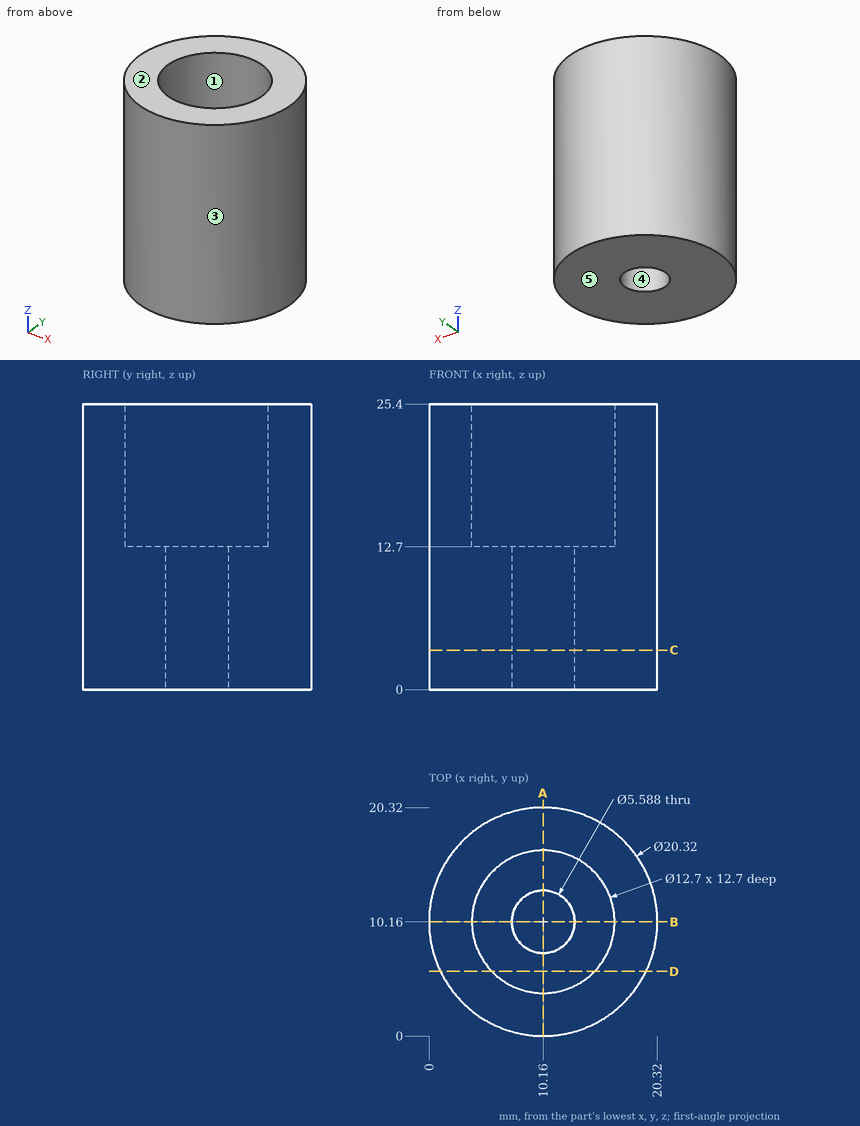
Part print with two shaded views. Sizes in mm from the minimum x, y, z corner. A direction names the side the tool comes from. Coordinates: 2 decimals unless noted, no trailing zeros. Write each loop counter-clockwise with the first axis right and the second up, starting at its lowest first coordinate (ties: lowest second). Pieces come first, ordered by that corner, then holes.
(1) Drill centre lines: line 1 (Y direction, x = 10.16, z = 22.5); line 2 (Y direction, x = 10.16, z = 3.25); line 3 (X direction, y = 10.5, z = 4.25). Where is each one in solid material? Low to high.
(2) Pin check, flat tips, straight feed: pin 1 Ø3 at (x, z) = (16.5, 13) entering from -Y; pin 2 Ø3.5 at (x, y) = (10.16, 10.16) entering from -Z; pin 3 Ø12 at (x, y) = (9.5, 14) entering from +Z; pin 4 Ø3 at (x, z) = (17, 11.5) entering from +Y. Stop position of each tip, or through.
(3) Cut at C-C on z = 3.5. List the corners of the cut face in (x, y), and give its area (3 significant figures).
(4) 3-axis set-ups, long thin cutter, end or side, ignore diameter. For the marked faces 1 and 2: which of +Z, -Z, +X, -X, +Y, -Y reach the whole face in a straight line?
(5) Cut at A-A on x = 10.16. List the corners of the cut face in (y, z).
(6) Mould opens along X. For the marked faces 3, 4 and 5 say: pulls with the +X half, pulls with the -X half, needs draft (parallel to the pull), parting line crosses it, or undercut.
(7) Cut at D-D on y = 5.75. List the corners of the cut face in (x, z), and give its area (3 significant figures).
Working result:
1. line 1: y = 0 to 3.81, 16.51 to 20.32
1. line 2: y = 0 to 7.37, 12.95 to 20.32
1. line 3: x = 0.01 to 7.39, 12.93 to 20.31
2. pin 1: stops at y = 1.23
2. pin 2: passes through
2. pin 3: stops at z = 25.4
2. pin 4: stops at y = 18.8
3. outline: circle Ø20.32 at (10.16, 10.16); hole circle Ø5.59 at (10.16, 10.16)
3. area: 300 mm2
4. face 1: +Z
4. face 2: +Z, +X, -X, +Y, -Y
5. outline: (0, 0) - (7.37, 0) - (7.37, 12.7) - (3.81, 12.7) - (3.81, 25.4) - (0, 25.4) - close; (12.95, 0) - (20.32, 0) - (20.32, 25.4) - (16.51, 25.4) - (16.51, 12.7) - (12.95, 12.7) - close
6. face 3: parting line crosses it
6. face 4: undercut
6. face 5: needs draft
7. outline: (1.01, 0) - (19.31, 0) - (19.31, 25.4) - (14.73, 25.4) - (14.73, 12.7) - (5.59, 12.7) - (5.59, 25.4) - (1.01, 25.4) - close
7. area: 349 mm2
